Source: CAD feature listing. Evaluate the final solid. Frame: model axes, mm. Face numbers are marked on the shaded views. Give positions to 0.01 mm unless a question says otherwise; leave off trailing zeros. Order: outer loops, then holes, each group sorted by start corner. A loop starts at its lowest first (then second) coordinate and runs counter-clockwise, first axis right, second up. Notation, with made-up numbers: (24.25, -8.5) -> (76.25, -8.5) arc R23 cw to (76.25, 11.5) -> close; hole circle Ø6 at (-40, 8). An arc over 180 degrees is marked (long way). Answer in a Markdown table with one row per item.
Autodesk Inventor part; units mm, degrees
ref_plane "YZ Plane" through (0, 0, 0) normal (1, 0, 0) x (0, 1, 0)
ref_plane "XZ Plane" through (0, 0, 0) normal (0, 1, 0) x (-1, 0, 0)
ref_plane "XY Plane" through (0, 0, 0) normal (0, 0, 1) x (1, 0, 0)
sketch "Sketch1" plane through (0, 0, 0) normal (0, 0, 1) x (1, 0, 0)
  line L0 (-21.15, -21.15) -> (21.15, -21.15)
  line L1 (21.15, -21.15) -> (21.15, 21.15)
  line L2 (21.15, 21.15) -> (-21.15, 21.15)
  line L3 (-21.15, 21.15) -> (-21.15, -21.15)
  line L4 (-21.15, -21.15) -> (21.15, 21.15) construction
  line L5 (21.15, -21.15) -> (-21.15, 21.15) construction
  line L6 (-15.5, -15.5) -> (15.5, -15.5) construction
  line L7 (15.5, -15.5) -> (15.5, 15.5) construction
  line L8 (15.5, 15.5) -> (-15.5, 15.5) construction
  line L9 (-15.5, 15.5) -> (-15.5, -15.5) construction
  line L10 (-15.5, -15.5) -> (15.5, 15.5) construction
  line L11 (15.5, -15.5) -> (-15.5, 15.5) construction
  circle A0 centre (-15.5, 15.5) radius 1.5
  circle A1 centre (15.5, 15.5) radius 1.5
  circle A2 centre (15.5, -15.5) radius 1.5
  circle A3 centre (-15.5, -15.5) radius 1.5
  point P0 (0, 0)
  dimension "d0" = 42.3
  dimension "d1" = 31
  dimension "d2" = 3
extrude "Extrusion1" add sketch "Sketch1" along normal blind 9
chamfer "Chamfer1" distance 4 angle 45 4 edges at (21.15, 21.15, 4.5) (21.15, -21.15, 4.5) (-21.15, 21.15, 4.5) (-21.15, -21.15, 4.5)
sketch "Sketch3" plane through (0, 0, 0) normal (0, 0, -1) x (-1, 0, 0)
  circle A0 centre (15.5, 15.5) radius 1.5
  line L0 (21.15, 17.15) -> (21.15, -17.15)
  line L1 (17.15, 21.15) -> (21.15, 17.15)
  line L2 (-17.15, 21.15) -> (17.15, 21.15)
  line L3 (-21.15, 17.15) -> (-17.15, 21.15)
  line L4 (-21.15, -17.15) -> (-21.15, 17.15)
  circle A1 centre (15.5, -15.5) radius 1.5
  circle A2 centre (-15.5, -15.5) radius 1.5
  circle A3 centre (-15.5, 15.5) radius 1.5
  circle A4 centre (15.5, 15.5) radius 1.5
  line L5 (21.15, -17.15) -> (17.15, -21.15)
  line L6 (21.15, 17.15) -> (21.15, -17.15)
  line L7 (17.15, 21.15) -> (21.15, 17.15)
  line L8 (-17.15, 21.15) -> (17.15, 21.15)
  line L9 (-21.15, 17.15) -> (-17.15, 21.15)
  line L10 (-21.15, -17.15) -> (-21.15, 17.15)
  line L11 (-17.15, -21.15) -> (-21.15, -17.15)
  line L12 (17.15, -21.15) -> (-17.15, -21.15)
  line L13 (-20.65, 16.9429) -> (-16.9429, 20.65)
  line L14 (-16.9429, 20.65) -> (16.9429, 20.65)
  line L15 (16.9429, 20.65) -> (20.65, 16.9429)
  line L16 (20.65, 16.9429) -> (20.65, -16.9429)
  line L17 (20.65, -16.9429) -> (16.9429, -20.65)
  line L18 (16.9429, -20.65) -> (-16.9429, -20.65)
  line L19 (-16.9429, -20.65) -> (-20.65, -16.9429)
  line L20 (-20.65, -16.9429) -> (-20.65, 16.9429)
  point P0 (0, 0)
  dimension "d8" = 0.5
  dimension "d10" = 0.5
  dimension "d11" = 0.5
  dimension "d12" = 0.5
extrude "Extrusion2" add sketch "Sketch3" along normal blind 20 contours A0 | A1 | A2 | A3 | L13 L14 L15 L16 L17 L18 L19 L20
sketch "Sketch4" plane through (0, 0, -20) normal (0, 0, -1) x (-1, 0, 0)
  line L0 (-21.15, 17.15) -> (-17.15, 21.15)
  line L1 (-17.15, 21.15) -> (17.15, 21.15)
  line L2 (17.15, 21.15) -> (21.15, 17.15)
  line L3 (21.15, 17.15) -> (21.15, -17.15)
  line L4 (21.15, -17.15) -> (17.15, -21.15)
  line L5 (17.15, -21.15) -> (-17.15, -21.15)
  line L6 (-17.15, -21.15) -> (-21.15, -17.15)
  line L7 (-21.15, -17.15) -> (-21.15, 17.15)
  point P0 (0, 0)
extrude "Extrusion3" add sketch "Sketch4" along normal blind 9
sketch "Sketch5" plane through (0, 0, 9) normal (0, 0, 1) x (1, 0, 0)
  circle A0 centre (0, 0) radius 11
  dimension "d17" = 22
extrude "Extrusion4" add sketch "Sketch5" along normal blind 1
sketch "Sketch6" plane through (0, 0, 10) normal (0, 0, 1) x (1, 0, 0)
  circle A0 centre (0, 0) radius 11
  circle A1 centre (0, 0) radius 4
  dimension "d20" = 8
extrude "Extrusion5" add sketch "Sketch6" along normal blind 210 contours A1
equation "\"d10\" = d8"
equation "\"d11\" = d8"
equation "\"d12\" = d8"
properties part number "StepperDrive-210mm"
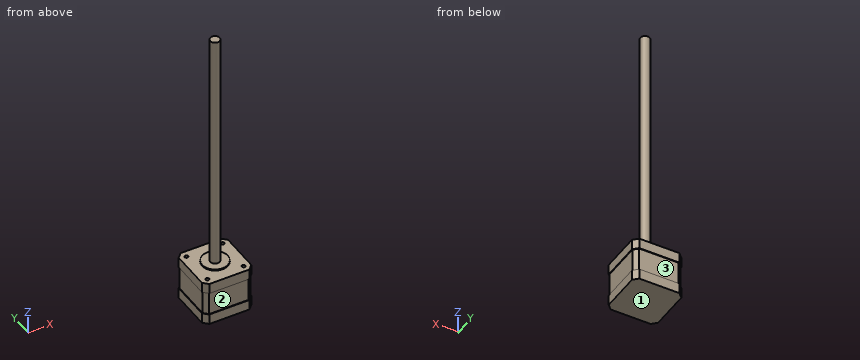
(1) Pull-direction query (Z, two-part tool) for the marked faces 1, 2 and 3; classes: +Z half, -Z half, draft (parallel to the pull), parting line (faces both ways), or undercut.
A:
| item | result |
|---|---|
| face 1 | -Z half |
| face 2 | undercut |
| face 3 | undercut |
(2) First-contact query: pin 1 Ø10 at (x, y) = (11, -11.5) entering from +Z; pin 2 Ø3.5 at (x, y) = (15, 15.5) entering from +Z; pin 3 Ø2 at (y, z) = (6, 103) entering from -X; pin 4 Ø0.9 at (x, y) = (15.5, -16) entering from +Z. Flat tips, straight axial feed; report the tip coordinate or a pass-through.
A:
| item | result |
|---|---|
| pin 1 | stops at z = 10 |
| pin 2 | stops at z = 9 |
| pin 3 | passes through |
| pin 4 | stops at z = 0 |
(3) Section query B-B (x = 0). Return the cut outline in (y, z), plus the area to 3 significant figures.
A:
| item | result |
|---|---|
| outline | (-21.15, -29) -> (21.15, -29) -> (21.15, -20) -> (20.65, -20) -> (20.65, 0) -> (21.15, 0) -> (21.15, 9) -> (11, 9) -> (11, 10) -> (4, 10) -> (4, 220) -> (-4, 220) -> (-4, 10) -> (-11, 10) -> (-11, 9) -> (-21.15, 9) -> (-21.15, 0) -> (-20.65, 0) -> (-20.65, -20) -> (-21.15, -20) -> close |
| area | 3,290 mm^2 |
(4) Ray query, probe 1 along X at (y, z) = (-15, 7); probe 2 along Y at (x, z) = (-15.5, 6.5). Return the intervals inside material, ascending.
A:
| item | result |
|---|---|
| probe 1 | x = -21.15 to -16.91, -14.09 to 14.09, 16.91 to 21.15 |
| probe 2 | y = -21.15 to -17, -14 to 14, 17 to 21.15 |
(5) Section query A-A (z = -5.5). Return the cut outline in (x, y), plus the area to 3 significant figures.
A:
| item | result |
|---|---|
| outline | (-20.65, -16.94) -> (-16.94, -20.65) -> (16.94, -20.65) -> (20.65, -16.94) -> (20.65, 16.94) -> (16.94, 20.65) -> (-16.94, 20.65) -> (-20.65, 16.94) -> close |
| area | 1,680 mm^2 |
(6) Section query C-C (y = 6.5). Return the cut outline in (x, z).
A:
| item | result |
|---|---|
| outline | (-21.15, -29) -> (21.15, -29) -> (21.15, -20) -> (20.65, -20) -> (20.65, 0) -> (21.15, 0) -> (21.15, 9) -> (8.87, 9) -> (8.87, 10) -> (-8.87, 10) -> (-8.87, 9) -> (-21.15, 9) -> (-21.15, 0) -> (-20.65, 0) -> (-20.65, -20) -> (-21.15, -20) -> close |
(7) Section query D-D (z = 96.5). Return the cut outline in (x, y), plus the area to 3 significant figures.
A:
| item | result |
|---|---|
| outline | circle Ø8 at (0, 0) |
| area | 50.3 mm^2 |
